Model file for the job. Use its own axes, mm. A direction names the side the tool comes from. Coordinates: 2 decimals unless noted, no trailing zeros. Write each loop counter-clockwise with the first axis right and the second up, starting at its lowest first coordinate (ties: lowest second). Pieces come first, ordered by that corner, then holes. Notation, with made-up numbers: M 46.25,68.5 L 55.25,68.5 A17 cw 55.25,79.5 Z; hole C 63.25,-18.75 d1. An arc over 180 degrees is marked long. Put each result on its own line as item: value. Start each with the question number.
Q1. Drill centre lines: line 1 along X through (y, z) = (-58, 3); line 2 along Z through (x, y) = (59, -27.5); line 3 along Z through (x, y) = (-36.5, -1). Where is each one in solid material? Low to high.
Q2. Cut at D-D (y = -50.8). Write the cut outline in (x, z).
Q3. Drop flat-ended pins along their axis: pin 1 (5 mm diameter, centred on x = -7, y = -20.5, fed in from +Z); pin 2 (4.5 mm diameter, centred on x = -37.975, z = 9, fed in from -Y); pin 3 (4 mm diameter, centred on y = 34, z = 14, fed in from -X). Give the stop position or say it passes through.
Q4. Cut at A-A (x = 57.75). Write the cut outline in (y, z), then the cut area to 3 significant figures.
Q5. Cut at B-B (y = -5). Give the number of separate pieces and of enclosed holes in the cut face, then the cut area to 4 significant figures.
Q6. Which spindle directions (+Z, -Z, +X, -X, +Y, -Y) get a long thin tool onto all of the face, cutting with end or side? Do faces 1 (the flat face through (-23.7, 36, 9)), 2 (the flat face through (-52.25, -24, 4)), 3 (the cylindrical face through (-54.278, 4.542, 69.148)), 4 (the flat face through (52.25, 53, 2)), 5 (the flat face through (-38, -34, 6)). Say none if no direction does.
Q7. Pull direction Y, two halves, no side cores. Call faces 6 (the flat face through (0, -18, 2)), 7 (the flat face through (-52.25, 24, 4)), 8 (the flat face through (79, 68, 2)): pulls with the +Y half, pulls with the -Y half, needs draft (parallel to the pull), parting line crosses it, or undercut.
Q8. Cut at C-C (y = 12.5). Write the cut outline in (x, z), then the cut area to 4 significant figures.
Autodesk Inventor part; units mm, degrees
ref_plane "YZ Plane" through (0, 0, 0) normal (1, 0, 0) x (0, 1, 0)
ref_plane "XZ Plane" through (0, 0, 0) normal (0, 1, 0) x (-1, 0, 0)
ref_plane "XY Plane" through (0, 0, 0) normal (0, 0, 1) x (1, 0, 0)
sketch "Эскиз1" plane through (0, 0, 0) normal (0, 0, 1) x (1, 0, 0)
  line L0 (-42.5, -28.25) -> (42.5, -28.25) construction
  line L1 (42.5, -28.25) -> (42.5, 28.25) construction
  line L2 (42.5, 28.25) -> (-42.5, 28.25) construction
  line L3 (-42.5, 28.25) -> (-42.5, -28.25) construction
  line L4 (-52.25, 38) -> (52.25, 38)
  line L5 (52.25, 38) -> (52.25, -38)
  line L6 (52.25, -38) -> (-52.25, -38)
  line L7 (-52.25, -38) -> (-52.25, 38)
  line L8 (52.25, 38) -> (52.25, 68) construction
  line L9 (52.25, 68) -> (105.25, 68) construction
  line L10 (105.25, 68) -> (105.25, 0) construction
  line L11 (105.25, 0) -> (105.25, -68) construction
  line L12 (105.25, -68) -> (52.25, -68) construction
  line L13 (52.25, -68) -> (52.25, 0) construction
  line L14 (52.25, 38) -> (52.25, 68)
  line L15 (105.25, 68) -> (52.25, 68)
  line L16 (105.25, 68) -> (105.25, -68)
  line L17 (105.25, -68) -> (52.25, -68)
  line L18 (52.25, -68) -> (52.25, 0)
  line L19 (-42.5, -28.25) -> (42.5, -28.25)
  line L20 (42.5, 28.25) -> (42.5, -28.25)
  line L21 (-42.5, -28.25) -> (-42.5, 28.25)
  line L22 (42.5, 28.25) -> (-42.5, 28.25)
  dimension "d0" = 85
  dimension "d1" = 56.5
  dimension "d2" = 9.75
  dimension "d3" = 68
  dimension "d4" = 53
  dimension "d5" = 68
extrude "Выдавливание1" add sketch "Эскиз1" along normal blind 5 contours L4 L5 L6 L7 | L14 L15 L16 L17 L18 L5 | L21 L22 L20 L19
sketch "Эскиз4" plane through (0, 0, 5) normal (0, 0, 1) x (1, 0, 0)
  line L0 (-42.5, -28.25) -> (42.5, -28.25) construction
  line L1 (-42.5, -28.25) -> (-42.5, 28.25)
  line L2 (42.5, 28.25) -> (-42.5, 28.25) construction
  line L3 (-42.5, 28.25) -> (42.5, 28.25)
  line L4 (42.5, 28.25) -> (42.5, -28.25)
  line L5 (42.5, -28.25) -> (-42.5, -28.25)
  line L6 (-42.5, -28.25) -> (-42.5, 28.25)
  point P0 (0, 0)
extrude "Выдавливание3" cut sketch "Эскиз4" against normal blind 1
sketch "Эскиз5" plane through (0, 0, 4) normal (0, 0, 1) x (1, 0, 0)
  line L0 (42.5, 28.25) -> (42.5, -28.25)
  line L1 (-42.5, 28.25) -> (42.5, 28.25)
  line L2 (-42.5, -28.25) -> (-42.5, 28.25)
  line L3 (42.5, -28.25) -> (-42.5, -28.25)
  line L4 (32.25, 18) -> (32.25, -18)
  line L5 (32.25, -18) -> (-32.25, -18)
  line L6 (-32.25, -18) -> (-32.25, 18)
  line L7 (-32.25, 18) -> (32.25, 18)
  point P0 (0, 0)
  dimension "d12" = 10.25
extrude "Выдавливание4" cut sketch "Эскиз5" against normal blind 8 contours L4 L5 L6 L7
sketch "Эскиз6" plane through (0, 0, 5) normal (0, 0, 1) x (1, 0, 0)
  line L0 (-33.05, 26.6205) -> (33.05, 26.6205) construction
  line L1 (33.05, 26.6205) -> (33.05, -26.6205) construction
  line L2 (33.05, -26.6205) -> (-33.05, -26.6205) construction
  line L3 (-33.05, -26.6205) -> (-33.05, 26.6205) construction
  line L4 (-33.05, 26.6205) -> (33.05, -26.6205) construction
  line L5 (33.05, 26.6205) -> (-33.05, -26.6205) construction
  point P0 (0, 0)
  dimension "d15" = 66.1
  dimension "d16" = 53.241
sketch "Эскиз7" plane through (0, 0, 5) normal (0, 0, 1) x (1, 0, 0)
  line L0 (-52.25, 38) -> (-52.25, -38) construction
  line L1 (-52.25, 0) -> (-56.25, 0)
  line L2 (-56.25, 10) -> (-52.25, 10)
  line L3 (-52.25, 10) -> (-52.25, -10)
  line L4 (-52.25, -10) -> (-56.25, -10)
  line L5 (-56.25, -10) -> (-56.25, 10)
  line L6 (-56.25, 10) -> (-52.25, -10) construction
  line L7 (-52.25, 10) -> (-56.25, -10) construction
  point P0 (0, 0)
  point P1 (-54.25, 0)
  dimension "d17" = 4
  dimension "d18" = 20
extrude "Выдавливание5" add sketch "Эскиз7" along normal blind 75 and the other way blind 5
sketch "Эскиз8" plane through (-56.25, -10, 80) normal (-1, 0, 0) x (0, 0, 1)
  line L0 (0, 0) -> (-80, 0)
  line L1 (0, 20) -> (0, 0)
  line L2 (-80, 20) -> (0, 20)
  line L3 (-80, 0) -> (-80, 20)
  line L4 (-80, 0) -> (-33.989, 0) construction
  line L5 (0, 0) -> (-80, 0) construction
  line L6 (-33.989, 0) -> (-33.989, 20) construction
  line L7 (0, 20) -> (-75, 20) construction
  line L8 (-33.989, 20) -> (-27.805, 20) construction
  line L9 (-27.805, 20) -> (-27.805, 14.454) construction
  circle A0 centre (-27.805, 14.454) radius 2
  line L10 (-27.805, 14.454) -> (-21.488, 14.454) construction
  line L11 (-27.805, 14.454) -> (-27.805, 5) construction
  circle A1 centre (-27.805, 5) radius 2
  circle A2 centre (-21.488, 14.454) radius 2
  circle A3 centre (-21.488, 5) radius 2
  circle A4 centre (-15.171, 14.454) radius 2
  circle A5 centre (-15.171, 5) radius 2
  circle A6 centre (-8.854, 14.454) radius 2
  circle A7 centre (-8.854, 5) radius 2
  point P0 (-80, 10)
  dimension "d23" = 46.011
  dimension "d24" = 6.184
  dimension "d25" = 5.546
  dimension "d26" = 4
  dimension "d27" = 6.317
  dimension "d28" = 9.454
  dimension "d29" = 4
  dimension "d32" = 6.317
extrude "Выдавливание6" cut sketch "Эскиз8" against normal blind 75 contours A0 | A1 | A2 | A3 | A4 | A5 | A6 | A7
sketch "Эскиз9" plane through (0, 0, 0) normal (0, 0, -1) x (-1, 0, 0)
  line L0 (-32.25, 18) -> (32.25, 18)
  line L1 (32.25, 18) -> (32.25, -18)
  line L2 (32.25, -18) -> (-32.25, -18)
  line L3 (-32.25, -18) -> (-32.25, 18)
  line L4 (-52.25, 68) -> (-52.25, 38)
  line L5 (-105.25, 68) -> (-52.25, 68)
  line L6 (-105.25, -68) -> (-105.25, 68)
  line L7 (-52.25, -68) -> (-105.25, -68)
  line L8 (-52.25, -38) -> (-52.25, -68)
  line L9 (52.25, -38) -> (-52.25, -38)
  line L10 (52.25, -10) -> (52.25, -38)
  line L11 (52.25, -10) -> (56.25, -10)
  line L12 (56.25, -10) -> (56.25, 10)
  line L13 (56.25, 10) -> (52.25, 10)
  line L14 (52.25, 38) -> (52.25, 10)
  line L15 (-52.25, 38) -> (52.25, 38)
  line L16 (52.25, -38) -> (52.25, -42) construction
  line L17 (52.25, -38) -> (-52.25, -38)
  line L18 (52.25, -38) -> (23.7, -38)
  line L19 (4.7, -38) -> (-23.85, -38)
  line L20 (56.25, 0) -> (0, 0) construction
  line L21 (52.25, 38) -> (-52.25, 38)
  line L22 (52.25, 38) -> (52.25, 42) construction
  line L23 (4.7, 38) -> (-23.85, 38)
  line L24 (23.7, 34) -> (52.25, 34)
  line L25 (23.7, 38) -> (23.7, 34)
  line L26 (52.25, 38) -> (52.25, 34) construction
  line L27 (52.25, 34) -> (52.25, 38)
  line L28 (4.7, 34) -> (4.7, 38)
  line L29 (-23.85, 34) -> (4.7, 34)
  line L30 (-23.85, 38) -> (-23.85, 34)
  line L31 (52.25, -38) -> (52.25, -34) construction
  line L32 (23.7, -38) -> (23.7, -34)
  line L33 (23.7, -34) -> (52.25, -34)
  line L34 (52.25, -34) -> (52.25, -38)
  line L35 (-23.85, -38) -> (-23.85, -34)
  line L36 (-23.85, -34) -> (4.7, -34)
  line L37 (4.7, -34) -> (4.7, -38)
  line L38 (52.25, 34) -> (23.7, 34)
  line L39 (23.7, 34) -> (23.7, 38)
  line L40 (23.7, 38) -> (52.25, 38)
  line L41 (52.25, 38) -> (52.25, 34)
  line L42 (4.7, 34) -> (-23.85, 34)
  line L43 (-23.85, 34) -> (-23.85, 38)
  line L44 (-23.85, 38) -> (4.7, 38)
  line L45 (4.7, 38) -> (4.7, 34)
  dimension "d39" = 4
extrude "Выдавливание7" add sketch "Эскиз9" against normal blind 13 contours L15 L28 L29 L30 | L15 L14 L24 L25 | L35 L36 L37 L9 | L32 L33 L10 L9
sketch "Эскиз10" plane through (-52.25, 38, 0) normal (0, 1, 0) x (1, 0, 0)
  line L0 (47.55, -5) -> (28.55, -5) construction
  line L1 (28.55, -5) -> (0, -5) construction
  line L2 (0, 0) -> (0, -13) construction
  line L3 (0, -5) -> (0, -13) construction
  line L4 (0, -13) -> (0, -5) construction
  circle A0 centre (14.275, -9) radius 2
  line L5 (38.05, -7) -> (38.05, -12) construction
  circle A1 centre (61.825, -9) radius 2
  point P0 (52.25, 0)
  dimension "d45" = 4
extrude "Выдавливание8" cut sketch "Эскиз10" against normal up to surface (76 mm away)
sketch "Эскиз11" plane through (0, 0, 5) normal (0, 0, 1) x (1, 0, 0)
  line L0 (-42.5, 28.25) -> (42.5, 28.25)
  line L1 (42.5, 28.25) -> (42.5, -28.25)
  line L2 (42.5, -28.25) -> (-42.5, -28.25)
  line L3 (-42.5, -28.25) -> (-42.5, 28.25)
  line L4 (-23.7, 38) -> (-23.7, 34)
  line L5 (-23.7, 34) -> (-52.25, 34)
  line L6 (-52.25, 34) -> (-52.25, 10)
  line L7 (-52.25, 10) -> (-52.25, -10)
  line L8 (-52.25, -10) -> (-52.25, -34)
  line L9 (-52.25, -34) -> (-23.7, -34)
  line L10 (-23.7, -34) -> (-23.7, -38)
  line L11 (-23.7, -38) -> (-4.7, -38)
  line L12 (-4.7, -38) -> (-4.7, -34)
  line L13 (-4.7, -34) -> (23.85, -34)
  line L14 (23.85, -34) -> (23.85, -38)
  line L15 (23.85, -38) -> (52.25, -38)
  line L16 (52.25, -38) -> (52.25, -68)
  line L17 (52.25, -68) -> (105.25, -68)
  line L18 (105.25, -68) -> (105.25, 68)
  line L19 (105.25, 68) -> (52.25, 68)
  line L20 (52.25, 68) -> (52.25, 38)
  line L21 (52.25, 38) -> (23.85, 38)
  line L22 (23.85, 38) -> (23.85, 34)
  line L23 (23.85, 34) -> (-4.7, 34)
  line L24 (-4.7, 34) -> (-4.7, 38)
  line L25 (-4.7, 38) -> (-23.7, 38)
  line L26 (52.25, -38) -> (52.25, -68)
  line L27 (52.25, -68) -> (57.75, -68)
  line L28 (52.25, -68) -> (105.25, -68)
  line L29 (57.75, -68) -> (57.75, -38) construction
  line L30 (23.85, -38) -> (52.25, -38)
  line L31 (57.75, -38) -> (52.25, -38) construction
  line L32 (57.75, -68) -> (57.75, -58.3)
  circle A0 centre (57.75, -58.3) radius 2
  line L33 (57.75, -58.3) -> (57.75, -50.8) construction
  circle A1 centre (57.75, -50.8) radius 2
  circle A2 centre (57.75, -43.3) radius 2
  line L34 (52.25, -68) -> (105.25, -68) construction
  line L35 (78.75, -68) -> (78.75, -28.25) construction
  circle A3 centre (99.75, -58.3) radius 2
  circle A4 centre (99.75, -50.8) radius 2
  circle A5 centre (99.75, -43.3) radius 2
  line L36 (105.25, -68) -> (105.25, 68) construction
  line L37 (105.25, 0) -> (77, 0) construction
  circle A6 centre (57.75, 58.3) radius 2
  circle A7 centre (57.75, 50.8) radius 2
  circle A8 centre (57.75, 43.3) radius 2
  circle A9 centre (99.75, 58.3) radius 2
  circle A10 centre (99.75, 50.8) radius 2
  circle A11 centre (99.75, 43.3) radius 2
  point P0 (0, 0)
  dimension "d48" = 5.5
  dimension "d49" = 9.7
  dimension "d50" = 4
  dimension "d51" = 7.5
  dimension "d54" = 7.5
extrude "Выдавливание9" cut sketch "Эскиз11" against normal blind 10 contours A0 | A1 | A2 | A3 | A4 | A5 | A6 | A7 | A8 | A9 | A10 | A11
properties part number "LIner"
Computed values:
1. line 1: 52.25 to 55.77, 59.73 to 97.77, 101.73 to 105.25
1. line 2: 0 to 5
1. line 3: 0 to 4
2. outline: M 52.25,0 L 55.75,0 L 55.75,5 L 52.25,5 Z; M 59.75,0 L 97.75,0 L 97.75,5 L 59.75,5 Z; M 101.75,0 L 105.25,0 L 105.25,5 L 101.75,5 Z
3. pin 1: z = 4
3. pin 2: y = -38
3. pin 3: x = -52.25
4. outline: M -68,0 L -60.3,0 L -60.3,5 L -68,5 Z; M -56.3,0 L -52.8,0 L -52.8,5 L -56.3,5 Z; M -48.8,0 L -45.3,0 L -45.3,5 L -48.8,5 Z; M -41.3,0 L 41.3,0 L 41.3,5 L -41.3,5 Z; M 45.3,0 L 48.8,0 L 48.8,5 L 45.3,5 Z; M 52.8,0 L 56.3,0 L 56.3,5 L 52.8,5 Z; M 60.3,0 L 68,0 L 68,5 L 60.3,5 Z
4. area: 560 mm2
5. separate pieces: 6
5. enclosed holes: 0
5. area: 700.5 mm2
6. face 1: +Z, +Y, -Y
6. face 2: +Z, -Z, -X, -Y
6. face 3: +X, -X
6. face 4: +Z, -Z, -X, +Y
6. face 5: +Z, +X, -X
7. face 6: undercut
7. face 7: needs draft
7. face 8: pulls with the +Y half
8. outline: M -52.25,0 L -32.25,0 L -32.25,4 L -42.5,4 L -42.5,5 L -52.25,5 Z; M 32.25,0 L 105.25,0 L 105.25,5 L 42.5,5 L 42.5,4 L 32.25,4 Z
8. area: 444.5 mm2
